Autodesk Inventor part; units mm, degrees
ref_plane "YZ Plane" through (0, 0, 0) normal (1, 0, 0) x (0, 1, 0)
ref_plane "XZ Plane" through (0, 0, 0) normal (0, 1, 0) x (-1, 0, 0)
ref_plane "XY Plane" through (0, 0, 0) normal (0, 0, 1) x (1, 0, 0)
sketch "Sketch1" plane through (0, 0, 0) normal (0, 0, 1) x (1, 0, 0)
  circle A0 centre (0, 0) radius 38.1
  circle A1 centre (0, 0) radius 3.1
  line L0 (-2.75, 1.4309) -> (-2.75, -1.4309)
  line L1 (2.192, 2.192) -> (4.3841, 0)
  line L2 (4.3841, 0) -> (2.192, -2.192)
  dimension "d0" = 76.2
  dimension "d1" = 6.2
  dimension "d2" = 2.75
extrude "Extrusion1" add sketch "Sketch1" along normal blind 25 contours A0 | L0 A1 picked at (-2.8371, 0.2455)
sketch "Sketch3" plane through (0, 0, 25) normal (0, 0, 1) x (1, 0, 0)
  circle A0 centre (0, 0) radius 38.1
  line L0 (4.3841, 0) -> (2.192, -2.192)
  arc A1 (-2.75, -1.4309) -> (2.192, -2.192) centre (0, 0) ccw
  line L1 (-2.75, -1.4309) -> (-2.75, 1.4309)
  arc A2 (2.192, 2.192) -> (-2.75, 1.4309) centre (0, 0) ccw
  line L2 (2.192, 2.192) -> (4.3841, 0)
  line L3 (0, 0) -> (38.1, 0) construction
  circle A3 centre (0, 0) radius 7.1
  circle A4 centre (0, 0) radius 34.1
  circle A5 centre (0, 0) radius 3.1 construction
  circle A6 centre (27.3278, 10) radius 5
  circle A7 centre (27.3278, -10) radius 5
  line L4 (27.3278, 10) -> (27.3278, 0) construction
  line L5 (27.3278, -10) -> (27.3278, 0) construction
  circle A8 centre (8.2583, 6) radius 3.1078
  circle A9 centre (8.2583, -6) radius 3.1078
  line L6 (8.2583, 6) -> (8.2583, 0) construction
  line L7 (8.2583, -6) -> (8.2583, 0) construction
  arc A10 (7.5566, 2.9724) -> (29.5391, 5.5155) centre (14.9864, 35.0288) ccw
  arc A11 (29.5391, -5.5155) -> (7.5566, -2.9724) centre (14.9864, -35.0288) ccw
  circle A12 centre (17.9553, 22.9001) radius 5
  arc A13 (14.3737, 26.3889) -> (5.1621, 6.2682) centre (37.9454, 3.4284) ccw
  circle A14 centre (-1.0658, 29.0805) radius 5
  circle A15 centre (-16.2308, 24.1531) radius 5
  circle A16 centre (-27.9865, 7.9727) radius 5
  circle A17 centre (-27.9865, -7.9727) radius 5
  circle A18 centre (-16.2308, -24.1531) radius 5
  circle A19 centre (17.9553, -22.9001) radius 5
  circle A20 centre (-1.0658, -29.0805) radius 5
  circle A21 centre (-3.1544, 9.7082) radius 3.1078
  circle A22 centre (-10.2078, 0) radius 3.1078
  circle A23 centre (-3.1544, -9.7082) radius 3.1078
  arc A24 (-0.4919, 8.1053) -> (3.8825, 29.7977) centre (-28.6833, 25.0774) ccw
  arc A25 (5.1621, -6.2682) -> (14.3737, -26.3889) centre (37.9454, -3.4284) ccw
  arc A26 (3.8825, -29.7977) -> (-0.4919, -8.1053) centre (-28.6833, -25.0774) ccw
  arc A27 (-4.3662, -6.8464) -> (-20.6557, -21.8248) centre (8.4652, -37.1477) ccw
  arc A28 (-20.6557, 21.8248) -> (-4.3662, 6.8464) centre (8.4652, 37.1477) ccw
  arc A29 (-7.8606, 2.0369) -> (-27.1396, 12.9005) centre (-32.7137, -19.5301) ccw
  arc A30 (-27.1396, -12.9005) -> (-7.8606, -2.0369) centre (-32.7137, 19.5301) ccw
  line L8 (8.2583, 6) -> (-3.1544, 9.7082) construction
  line L9 (-3.1544, 9.7082) -> (-10.2078, 0) construction
  line L10 (-10.2078, 0) -> (-3.1544, -9.7082) construction
  line L11 (-3.1544, -9.7082) -> (8.2583, -6) construction
  line L12 (17.9553, 22.9001) -> (-1.0658, 29.0805) construction
  line L13 (-16.2308, 24.1531) -> (-27.9865, 7.9727) construction
  line L14 (-27.9865, -7.9727) -> (-16.2308, -24.1531) construction
  line L15 (-1.0658, -29.0805) -> (17.9553, -22.9001) construction
  point P0 (21.0404, -26.8349)
  point P1 (32.0233, -11.7182)
  point P2 (-19.0196, -28.3031)
  point P3 (-1.2489, -34.0771)
  point P4 (-32.7952, 9.3426)
  point P5 (-32.7952, -9.3426)
  point P6 (-1.2489, 34.0771)
  point P7 (-19.0196, 28.3031)
  point P8 (32.0233, 11.7182)
  point P9 (21.0404, 26.8349)
  dimension "d32" = 10
  dimension "d25" = 4
  dimension "d26" = 4
  dimension "d29" = 10
  dimension "d30" = 6
  dimension "d31" = 12
extrude "Extrusion4" cut sketch "Sketch3" against normal through all contours A8 | A9 | A21 | A13 A12 A4 A6 A10 A8 | A23 | A11 A7 A4 A19 A25 A9 | A22 | A28 A15 A4 A14 A24 A21 | A12 | A6 | A26 A20 A4 A18 A27 A23 | A7 | A19 | A22 A30 A17 A4 A16 A29 | A15 | A14 | A20 | A18 | A16 | A17
sketch "Sketch4" plane through (0, 0, 25) normal (0, 0, 1) x (1, 0, 0)
  arc A0 (-27.1396, 12.9005) -> (-32.7952, 9.3426) centre (-27.9865, 7.9727) ccw
  arc A1 (-7.8606, 2.0369) -> (-27.1396, 12.9005) centre (-32.7137, -19.5301) ccw
  arc A2 (-7.8606, -2.0369) -> (-7.8606, 2.0369) centre (-10.2078, 0) ccw
  arc A3 (-27.1396, -12.9005) -> (-7.8606, -2.0369) centre (-32.7137, 19.5301) ccw
  arc A4 (-32.7952, -9.3426) -> (-27.1396, -12.9005) centre (-27.9865, -7.9727) ccw
  arc A5 (-32.7952, 9.3426) -> (-32.7952, -9.3426) centre (0, 0) ccw
  arc A6 (3.8825, -29.7977) -> (-0.4919, -8.1053) centre (-28.6833, -25.0774) ccw
  arc A7 (-1.2489, -34.0771) -> (3.8825, -29.7977) centre (-1.0658, -29.0805) ccw
  arc A8 (-19.0196, -28.3031) -> (-1.2489, -34.0771) centre (0, 0) ccw
  arc A9 (-20.6557, -21.8248) -> (-19.0196, -28.3031) centre (-16.2308, -24.1531) ccw
  arc A10 (-4.3662, -6.8464) -> (-20.6557, -21.8248) centre (8.4652, -37.1477) ccw
  arc A11 (-0.4919, -8.1053) -> (-4.3662, -6.8464) centre (-3.1544, -9.7082) ccw
  arc A12 (-20.6557, 21.8248) -> (-4.3662, 6.8464) centre (8.4652, 37.1477) ccw
  arc A13 (-19.0196, 28.3031) -> (-20.6557, 21.8248) centre (-16.2308, 24.1531) ccw
  arc A14 (-1.2489, 34.0771) -> (-19.0196, 28.3031) centre (0, 0) ccw
  arc A15 (3.8825, 29.7977) -> (-1.2489, 34.0771) centre (-1.0658, 29.0805) ccw
  arc A16 (-0.4919, 8.1053) -> (3.8825, 29.7977) centre (-28.6833, 25.0774) ccw
  arc A17 (-4.3662, 6.8464) -> (-0.4919, 8.1053) centre (-3.1544, 9.7082) ccw
  arc A18 (29.5391, -5.5155) -> (7.5566, -2.9724) centre (14.9864, -35.0288) ccw
  arc A19 (32.0233, -11.7182) -> (29.5391, -5.5155) centre (27.3278, -10) ccw
  arc A20 (21.0404, -26.8349) -> (32.0233, -11.7182) centre (0, 0) ccw
  arc A21 (14.3737, -26.3889) -> (21.0404, -26.8349) centre (17.9553, -22.9001) ccw
  arc A22 (5.1621, -6.2682) -> (14.3737, -26.3889) centre (37.9454, -3.4284) ccw
  arc A23 (7.5566, -2.9724) -> (5.1621, -6.2682) centre (8.2583, -6) ccw
  arc A24 (7.5566, 2.9724) -> (29.5391, 5.5155) centre (14.9864, 35.0288) ccw
  arc A25 (5.1621, 6.2682) -> (7.5566, 2.9724) centre (8.2583, 6) ccw
  arc A26 (14.3737, 26.3889) -> (5.1621, 6.2682) centre (37.9454, 3.4284) ccw
  arc A27 (21.0404, 26.8349) -> (14.3737, 26.3889) centre (17.9553, 22.9001) ccw
  arc A28 (32.0233, 11.7182) -> (21.0404, 26.8349) centre (0, 0) ccw
  arc A29 (29.5391, 5.5155) -> (32.0233, 11.7182) centre (27.3278, 10) ccw
  circle A30 centre (0, 0) radius 38.1
  line L0 (4.3841, 0) -> (2.192, -2.192)
  arc A31 (-2.75, -1.4309) -> (2.192, -2.192) centre (0, 0) ccw
  line L1 (-2.75, -1.4309) -> (-2.75, 1.4309)
  arc A32 (2.192, 2.192) -> (-2.75, 1.4309) centre (0, 0) ccw
  line L2 (2.192, 2.192) -> (4.3841, 0)
  line L3 (37.8894, 4) -> (40.8894, 4)
  line L4 (40.8894, 4) -> (40.8894, -4)
  line L5 (40.8894, -4) -> (37.8894, -4)
  line L6 (37.8894, -4) -> (37.8894, 4)
  circle A33 centre (0, 0) radius 38.1
  point P0 (40.8894, 0)
  dimension "d41" = 8
  dimension "d42" = 3
extrude "Extrusion5" add sketch "Sketch4" against normal up to surface (25 mm away) contours A30 L3 L4 L5
pattern_circular "Circular Pattern2" count 12 over 360 about axis through (0, 0, 0) along (0, 0, 1) of "Extrusion5"
equation "\"d0\" = Wheel_Diameter"
equation "\"d1\" = Axel_Diamter"
equation "\"d3\" = Wheel_Thickness"
equation "\"Wheel_Diameter\" = 76.2"
equation "\"Axel_Diamter\" = 6.2"
equation "\"Axel_Cuttout_Dist\" = 2.75"
equation "\"Wheel_Thickness\" = 25"
equation "\"Tread_Height\" = 3"
equation "\"Tread_Width\" = 8"
properties part number "Drive_Wheel"
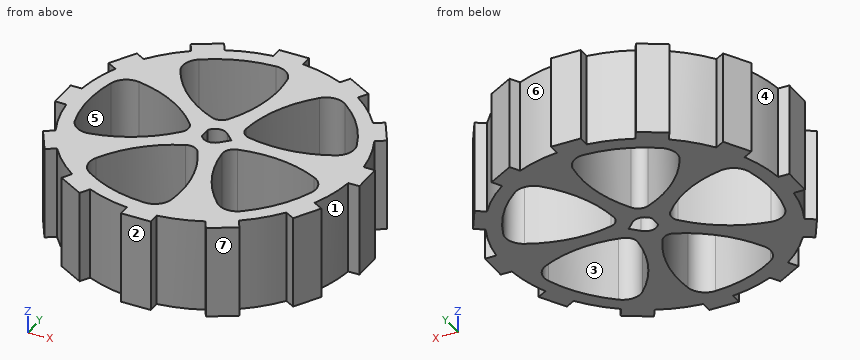
Read the model definition and answer for the solid it produces. Units are mm, in the model's axes. Face numbers are marked on the shaded views. A direction names the side the tool comes from. Give positions to 0.01 mm unless a question says otherwise; leave off trailing zeros. Loops run counter-clockwise (first coordinate to the right, second up) from the corner with the lowest first, then second, coordinate; pieces in that order, holes last. Notation, with made-up numbers: (-8, 74) -> (16, 74) arc R23 cw to (16, 106) -> close; hole circle Ø11 at (-13, -21.5). An arc over 180 degrees is marked (long way). Use a Markdown table: item, result.
Q1. Each of these flat-tipped pins is pushed along its axis until it touches: pin 1 (2.5 mm diameter, centred on y = -40, z = 12.5, fed in from -X); pin 2 (8 mm diameter, centred on y = 12.5, z = 21.5, fed in from -X); pin 3 (1.5 mm diameter, centred on y = 20, z = 22.5, fed in from -X); pin 4 (1.5 mm diameter, centred on x = 1, y = -31, fed in from +Z). Where does it stop, or does it pass through?
Solved:
| item | result |
|---|---|
| pin 1 | stops at x = -4 |
| pin 2 | stops at x = -37.14 |
| pin 3 | stops at x = -36.1 |
| pin 4 | passes through |
Q2. Section C-C, the plane y = 32 is taken. Determine the outline of the cut face in (x, z), then the cut area to 3 significant figures.
Solved:
| item | result |
|---|---|
| outline | (-23.09, 0) -> (-11.78, 0) -> (-11.78, 25) -> (-23.09, 25) -> close; (2.99, 0) -> (23.09, 0) -> (23.09, 25) -> (2.99, 25) -> close |
| area | 785 mm^2 |
Q3. Determine the mould class of the marked faces 4, 5, 6 and 7 for opening direction Y: pulls with the +Y half, pulls with the -Y half, needs draft (parallel to the pull), parting line crosses it, or undercut.
Solved:
| item | result |
|---|---|
| face 4 | undercut |
| face 5 | undercut |
| face 6 | pulls with the +Y half |
| face 7 | pulls with the -Y half |
Q4. A tool of negligible diameter and unlimited length cuts with its end or side. For the marked faces 1, 2 and 3, from which of +Z, -Z, +X, -X, +Y, -Y can it reach the whole face along a straight path? Write none if from no direction.
Solved:
| item | result |
|---|---|
| face 1 | +Z, -Z, +X |
| face 2 | +Z, -Z, +X, -X, -Y |
| face 3 | +Z, -Z |
Q5. Section A-A, the plane y = 20 is taken. Determine the outline of the cut face in (x, z).
Solved:
| item | result |
|---|---|
| outline | (-35.67, 0) -> (-19.62, 0) -> (-19.62, 25) -> (-35.67, 25) -> close; (3.83, 0) -> (9.52, 0) -> (9.52, 25) -> (3.83, 25) -> close; (27.62, 0) -> (35.67, 0) -> (35.67, 25) -> (27.62, 25) -> close |
Q6. Find the intervals of material crossed by line 1 along X through (y, z) = (-18.5, 19); line 2 along X through (y, z) = (22, 22.5); line 3 along Y through (x, z) = (-15.5, 14.5), in increasing order.
Solved:
| item | result |
|---|---|
| line 1 | x = -36.53 to -18.65, 3.56 to 8.69, 28.65 to 36.53 |
| line 2 | x = -34.51 to -20.74, 4.08 to 10.78, 26.05 to 34.51 |
| line 3 | y = -34.85 to -30.37, -14.6 to -8.51, 8.51 to 14.6, 30.37 to 34.85 |
Q7. Section B-B, the plane x = 25.5 is taken. Determine the outline of the cut face in (y, z).
Solved:
| item | result |
|---|---|
| outline | (-28.31, 0) -> (-22.64, 0) -> (-22.64, 25) -> (-28.31, 25) -> close; (-3.85, 0) -> (3.85, 0) -> (3.85, 25) -> (-3.85, 25) -> close; (22.64, 0) -> (28.31, 0) -> (28.31, 25) -> (22.64, 25) -> close |
Q8. Section D-D, the plane z = 22.25 is taken. Count the separate pieces of the cut face and the enclosed holes in it, then the cut area to 3 significant figures.
Solved:
| item | result |
|---|---|
| separate pieces | 1 |
| enclosed holes | 6 |
| area | 2,300 mm^2 |
